from build123d import *

# Parameters (mm, degrees)
SKETCH1_R           = 9.525
BOSS_EXTRUDE1_DEPTH = 2.54
SKETCH3_R           = 28.575
BOSS_EXTRUDE2_DEPTH = 12.7
CUT_EXTRUDE2_DEPTH  = 16.24
CUT_EXTRUDE3_DEPTH  = 8.466666667
SKETCH5_R           = 1.63195
CUT_EXTRUDE4_DEPTH  = 16.24


with BuildPart() as part:
    # Sketch1 → Boss-Extrude1 (new body)
    with BuildSketch(Plane(origin=(0, 0, 0), x_dir=(1, 0, 0), z_dir=(0, 1, 0))):
        Circle(SKETCH1_R)
    extrude(amount=BOSS_EXTRUDE1_DEPTH)

    # Sketch3 → Boss-Extrude2 (add)
    with BuildSketch(Plane(origin=(0, 2.54, 0), x_dir=(1, 0, 0), z_dir=(0, 1, 0))):
        Circle(SKETCH3_R)
        with BuildLine():
            Line((-2.465251405, 9.200443495), (-6.574003746, 24.534515988))
            ThreePointArc((-6.574003746, 24.534515988), (-17.960512242, 17.960512242), (-24.534515988, 6.574003746))
            Line((-24.534515988, 6.574003746), (-9.200443495, 2.465251405))
            ThreePointArc((-9.200443495, 2.465251405), (-6.735192091, 6.735192091), (-2.465251405, 9.200443495))
        make_face(mode=Mode.SUBTRACT)
        with BuildLine():
            Line((9.200443495, 2.465251405), (24.534515988, 6.574003746))
            ThreePointArc((24.534515988, 6.574003746), (17.960512242, 17.960512242), (6.574003746, 24.534515988))
            Line((6.574003746, 24.534515988), (2.465251405, 9.200443495))
            ThreePointArc((2.465251405, 9.200443495), (6.735192091, 6.735192091), (9.200443495, 2.465251405))
        make_face(mode=Mode.SUBTRACT)
        with BuildLine():
            Line((9.200443495, -2.465251405), (24.534515988, -6.574003746))
            ThreePointArc((24.534515988, -6.574003746), (17.960512242, -17.960512242), (6.574003746, -24.534515988))
            Line((6.574003746, -24.534515988), (2.465251405, -9.200443495))
            ThreePointArc((2.465251405, -9.200443495), (6.735192091, -6.735192091), (9.200443495, -2.465251405))
        make_face(mode=Mode.SUBTRACT)
        with BuildLine():
            Line((-9.200443495, -2.465251405), (-24.534515988, -6.574003746))
            ThreePointArc((-24.534515988, -6.574003746), (-17.960512242, -17.960512242), (-6.574003746, -24.534515988))
            Line((-6.574003746, -24.534515988), (-2.465251405, -9.200443495))
            ThreePointArc((-2.465251405, -9.200443495), (-6.735192091, -6.735192091), (-9.200443495, -2.465251405))
        make_face(mode=Mode.SUBTRACT)
    extrude(amount=BOSS_EXTRUDE2_DEPTH)

    # Sketch4 → Cut-Extrude2 (cut, through all)
    with BuildSketch(Plane(origin=(0, 15.24, 0), x_dir=(1, 0, 0), z_dir=(0, 1, 0))):
        with BuildLine():
            Line((12.604555768, 1.554082971), (25.196118384, 3.211793638))
            ThreePointArc((25.196118384, 3.211793638), (25.399675108, -0.128469484), (25.162340107, -3.466502611))
            Line((25.162340107, -3.466502611), (12.570536445, -1.80876021))
            ThreePointArc((12.570536445, -1.80876021), (12.699350202, -0.128469656), (12.604555768, 1.554082971))
        make_face()
        with BuildLine():
            Line((-12.604555768, 1.554082971), (-25.196118384, 3.211793638))
            ThreePointArc((-25.196118384, 3.211793638), (-25.399675108, -0.128469484), (-25.162340107, -3.466502611))
            Line((-25.162340107, -3.466502611), (-12.570536445, -1.80876021))
            ThreePointArc((-12.570536445, -1.80876021), (-12.699350202, -0.128469656), (-12.604555768, 1.554082971))
        make_face()
        with BuildLine():
            Line((1.554082971, 12.604555768), (3.211793638, 25.196118384))
            ThreePointArc((3.211793638, 25.196118384), (-0.128469484, 25.399675108), (-3.466502611, 25.162340107))
            Line((-3.466502611, 25.162340107), (-1.80876021, 12.570536445))
            ThreePointArc((-1.80876021, 12.570536445), (-0.128469656, 12.699350202), (1.554082971, 12.604555768))
        make_face()
        with BuildLine():
            Line((-1.80876021, -12.570536445), (-3.466502611, -25.162340107))
            ThreePointArc((-3.466502611, -25.162340107), (-0.128469484, -25.399675108), (3.211793638, -25.196118384))
            Line((3.211793638, -25.196118384), (1.554082971, -12.604555768))
            ThreePointArc((1.554082971, -12.604555768), (-0.128469656, -12.699350202), (-1.80876021, -12.570536445))
        make_face()
    extrude(amount=-CUT_EXTRUDE2_DEPTH, mode=Mode.SUBTRACT)

    # Sketch2 → Cut-Extrude3 (cut)
    with BuildSketch(Plane(origin=(0, 0, 0), x_dir=(1, 0, 0), z_dir=(0, 1, 0))):
        Polygon((-4.552853785, 1.885853785), (-1.885853785, 4.552853785), (0, 2.667), (1.885853785, 4.552853785), (4.552853785, 1.885853785), (2.667, 0), (4.552853785, -1.885853785), (1.885853785, -4.552853785), (0, -2.667), (-1.885853785, -4.552853785), (-4.552853785, -1.885853785), (-2.667, 0), align=None)
    extrude(amount=CUT_EXTRUDE3_DEPTH, mode=Mode.SUBTRACT)

    # Sketch5 → Cut-Extrude4 (cut, through all)
    with BuildSketch(Plane(origin=(0, 15.24, 0), x_dir=(1, 0, 0), z_dir=(0, 1, 0))):
        Circle(SKETCH5_R)
    extrude(amount=-CUT_EXTRUDE4_DEPTH, mode=Mode.SUBTRACT)


solid = part.part
CAD build for the part. Positions are in the model's coordinates, mm. A direction names the side the tool comes from. Give positions to 0.01 mm unless a question says otherwise; leave off trailing zeros. Write each loop counter-clockwise with the first axis right and the second up, starting at its lowest first coordinate (ties: lowest second). Pieces come first, ordered by that corner, then holes. Notation, with made-up numbers: M 10,33.25 L 52,33.25 A8 cw 52,40.25 Z; hole C 51.5,45.25 d6. An arc over 180 degrees is marked long. Put each result on its own line as item: value. Start each with the question number.
(1) Band-saw the part on D-D, the plane z = -21. Write the cut outline in (x, y), and give its area (3 significant figures).
(2) Band-saw the part on A-A, the plane z = 18.5. Write the cut outline in (x, y), and give its area (3 significant figures).
(3) Band-saw the part on B-B, the plane y = 14. Give the number of separate pieces and of enclosed holes in the cut face, and give its area (3 significant figures).
(4) Flat gauge pins, fed straight in: pin 1 Ø2 at (x, y) = (-2, 13) entering from +Z; pin 2 Ø3 at (x, y) = (11, 7.5) entering from +Z; pin 3 Ø2 at (x, z) = (22, -18.5) entering from +Y; pin 4 Ø6 at (x, z) = (2.5, -23) entering from -Y. Where does each tip first touch, or does it go through?
(5) Mould opens along Z. For faces 3 (the face through (-28.547, 8.801, -1.256)), 4 (the face through (4, 0, 0)), 5 (the face through (-2.65, 8.98, -18.95)) say: +Z half, -Z half, draft (parallel to the pull), parting line (faces both ways), or undercut.
(6) Probe L1, parallel to Z at x = 0, y = 12.25 (3 decimals); L2, parallel to X at y = 9.5, z = 18.5. List the from-to ranges inside material, lowest first.
(7) Which spindle directions (+Z, -Z, +X, -X, +Y, -Y) get a long thin tool onto all of the face, cutting with end or side? Do faces 1 (the face through (16.8, 8.8, 4.5)), 2 (the face through (-0.93, 4.174, 3.597)). Say none if no direction does.
Response values:
1. outline: M -19.38,2.54 L -14.29,2.54 L -14.29,15.24 L -19.38,15.24 Z; M -5.63,2.54 L -2.92,2.54 L -2.92,15.24 L -5.63,15.24 Z; M 2.66,2.54 L 5.63,2.54 L 5.63,15.24 L 2.66,15.24 Z; M 14.29,2.54 L 19.38,2.54 L 19.38,15.24 L 14.29,15.24 Z
1. area: 201 mm2
2. outline: M -21.78,2.54 L -17.4,2.54 L -17.4,15.24 L -21.78,15.24 Z; M -4.96,2.54 L -2.59,2.54 L -2.59,15.24 L -4.96,15.24 Z; M 2.33,2.54 L 4.96,2.54 L 4.96,15.24 L 2.33,15.24 Z; M 17.4,2.54 L 21.78,2.54 L 21.78,15.24 L 17.4,15.24 Z
2. area: 175 mm2
3. separate pieces: 1
3. enclosed holes: 9
3. area: 1,140 mm2
4. pin 1: stops at z = 28.56
4. pin 2: stops at z = 26.95
4. pin 3: stops at y = 15.24
4. pin 4: stops at y = 2.54
5. face 3: parting line
5. face 4: draft
5. face 5: undercut
6. L1: z = -28.575 to -25.4, -12.7 to -1.632, 1.632 to 12.7, 25.4 to 28.575
6. L2: x = -21.78 to -17.4, -4.96 to -2.59, 2.33 to 4.96, 17.4 to 21.78
7. face 1: +Y, -Y
7. face 2: -Y
